Part model, mm, in its own coordinate system. A direction names the side the tool comes from. Give positions to 0.01 mm unless a question says otherwise; leave off trailing zeros. Order: outer loops, then holes, each group sorted by start corner. A loop starts at its lowest first (then second) coordinate and runs counter-clockwise, first axis right, second up. Notation, with made-up numbers: (21.5, -16.5) - (28.5, -16.5) arc R16 ccw to (28.5, 11.5) - close; hole circle Ø7 at (-24.75, 29). An arc over 180 degrees is marked (long way). One line per item, written item: value.
```python
from build123d import *

# Parameters (mm, degrees)
BOX044_W     = 52
BOX044_H     = 15
BOX044_DEPTH = 5
FILLET008_R  = 2
BOX043_W     = 27.8
BOX043_H     = 15.15
BOX043_DEPTH = 2.4


with BuildPart() as fillet008:
    # Box044 → Box044 (new body)
    with BuildSketch(Plane(origin=(-4, 17.15, 0), x_dir=(1, 0, 0), z_dir=(0, 0, 1))):
        with Locations((26, 7.5)):
            Rectangle(BOX044_W, BOX044_H)
    extrude(amount=BOX044_DEPTH)

    # Fillet008
    fillet008_edges = [fillet008.edges().sort_by_distance(p)[0] for p in [
        (-4, 32.15, 2.5),
        (48, 32.15, 2.5),
    ]]
    fillet(fillet008_edges, radius=FILLET008_R)


with BuildPart() as exterior_parte2_v2:
    # Box043 → Box043 (new body)
    with BuildSketch(Plane(origin=(8.1, 2, 2.6), x_dir=(1, 0, 0), z_dir=(0, 0, 1))):
        with Locations((13.9, 7.575)):
            Rectangle(BOX043_W, BOX043_H)
    extrude(amount=BOX043_DEPTH)

    # Fusion023005: union Fillet008
    add(fillet008.part)


with BuildPart() as exterior_parte2_v2_1:
    # Fusion023005 placement: moved
    add(exterior_parte2_v2.part.moved(Location((0, -2, 0))))


solid = exterior_parte2_v2_1.part
```
1) Drill centre lines: line 1 along Y through (x, z) = (35, 1.7); line 2 along Z through (x, y) = (29, 13); line 3 along X through (y, z) = (11, 4.1). Where is each one in solid material? Low to high. Write a range as from..to.
Outcome:
line 1: y = 15.15..30.15
line 2: z = 2.6..5
line 3: x = 8.1..35.9
2) Cut at C-C, the plane y = 8. Give the cut face in (x, z), then the cut area to 3 significant figures.
Outcome:
outline: (8.1, 2.6) - (35.9, 2.6) - (35.9, 5) - (8.1, 5) - close
area: 66.7 mm^2
3) Which spindle directions (+Z, -Z, +X, -X, +Y, -Y) get a long thin tool onto all of the face, cutting with end or side? Do faces 1 (the flat face through (8.1, 7, 4)), 2 (the flat face through (35.9, 7, 4)), 3 (the flat face through (22, 8, 2.6)). Say none if no direction does.
Outcome:
face 1: +Z, -Z, -X, -Y
face 2: +Z, -Z, +X, -Y
face 3: -Z, +X, -X, -Y
4) Pin check, flat tips, straight feed: pin 1 (16.5 mm diameter, centred on x = 16.5, y = 11, fed in from -Z); pin 2 (1 mm diameter, centred on x = 19.5, y = 9, fed in from -Z); pin 3 (1 mm diameter, centred on x = 14, z = 1.5, fed in from -Y); pin 4 (1.5 mm diameter, centred on y = 11, z = 3, fed in from -X). Stop position of each tip, or through.
Outcome:
pin 1: stops at z = 0
pin 2: stops at z = 2.6
pin 3: stops at y = 15.15
pin 4: stops at x = 8.1
5) Cut at A-A, the plane x = 14.5. Give the cut face in (y, z), then the cut area to 3 significant figures.
Outcome:
outline: (0, 2.6) - (15.15, 2.6) - (15.15, 0) - (30.15, 0) - (30.15, 5) - (0, 5) - close
area: 111 mm^2
6) Cut at B-B, the plane z = 1.5. Give the cut face in (x, y).
Outcome:
outline: (-4, 15.15) - (48, 15.15) - (48, 28.15) arc R2 ccw to (46, 30.15) - (-2, 30.15) arc R2 ccw to (-4, 28.15) - close
7) Cut at D-D, the plane x = 2. Give the cut face in (y, z).
Outcome:
outline: (15.15, 0) - (30.15, 0) - (30.15, 5) - (15.15, 5) - close
